```python
from build123d import *

# Parameters (mm, degrees)
F0_W     = 19.05
F0_H     = 6.35
F1_DEPTH = 36.83


with BuildPart() as f1:
    # F0 (on Front) → F1 (new body)
    with BuildSketch(Plane.XZ):
        Polygon((-37.449954, 6.35), (-37.449954, 19.05), (-37.449954, 25.4), (-56.499954, 25.4), (-56.499954, 6.35), align=None)
        with Locations((-27.924954, 22.225)):
            Rectangle(F0_W, F0_H)
        Polygon((-37.449954, 0), (-18.399954, 0), (-18.399954, 19.05), (-37.449954, 19.05), (-37.449954, 6.35), align=None)
    extrude(amount=-F1_DEPTH)


solid = f1.part
```
Geometry check sheet. Reference: the model listing, model coordinates, mm. A direction names the side the tool comes from. Coordinates: 2 decimals unless noted, no trailing zeros. Order: outer loops, then holes, each group sorted by start corner. A loop starts at its lowest first (then second) coordinate and runs counter-clockwise, first axis right, second up. Notation, with made-up numbers: (-23, 14) - (-13, 14) arc R23 ccw to (-13, 24) - close; hole circle Ø10 at (77, 19.25). An arc over 180 degrees is marked (long way). Answer as a JSON object with one key per item and string values. Group by question number.
Item 1: Tool access check on faces 1 (the face through (-18.4, 18, 13)), 2 (the face through (-37.45, 18, 3)). Record the directions out of +Z, -Z, +X, -X, +Y, -Y that give a thin tool (end or side, any length) a straight path to the whole face; none if there is none.
Item 2: Scan lines: probe 1 along Z at (x, y) = (-40, 34); probe 2 along X at (y, z) = (18, 5.25). Record each from-to range of solid material in increasing order.
Item 3: Sectioned sample at C-C, the plane x = -47. Record the cut outline in (y, z), and give its area (3 significant figures).
Item 4: Sectioned sample at A-A, the plane y = 14. Record the cut outline in (x, z).
Item 5: Depth check by flat-ended pin: pin 1 Ø5.5 at (x, y) = (-47, 9.5) entering from -Z; pin 2 Ø1.9 at (y, z) = (25, 1.5) entering from -X. Enter the tip coordinate at first touch or a pass-through.
Item 6: Sectioned sample at B-B, the plane z = 4.5. Record the cut outline in (x, y).
Resolved:
{
 "1": {"face 1": "+Z, -Z, +X, +Y, -Y", "face 2": "-Z, -X, +Y, -Y"},
 "2": {"probe 1": "6.35 to 25.4", "probe 2": "-37.45 to -18.4"},
 "3": {"outline": "(0, 6.35) - (36.83, 6.35) - (36.83, 25.4) - (0, 25.4) - close", "area": "702 mm^2"},
 "4": {"outline": "(-56.5, 6.35) - (-37.45, 6.35) - (-37.45, 0) - (-18.4, 0) - (-18.4, 25.4) - (-56.5, 25.4) - close"},
 "5": {"pin 1": "z = 6.35", "pin 2": "x = -37.45"},
 "6": {"outline": "(-37.45, 0) - (-18.4, 0) - (-18.4, 36.83) - (-37.45, 36.83) - close"}
}
